from build123d import *

# Parameters (mm, degrees)
F1_DEPTH = 12.7
F3_DEPTH = 12.701


with BuildPart() as f1:
    # F0 (on Top) → F1 (new body)
    with BuildSketch(Plane.XY):
        with BuildLine():
            Line((-53.430256, 31.75), (-82.55, 31.75))
            ThreePointArc((-82.55, 31.75), (-87.040128, 29.890128), (-88.9, 25.4))
            Line((-88.9, 25.4), (-88.9, 15.330256))
            ThreePointArc((-88.9, 15.330256), (-88.416635, 12.900216), (-87.040128, 10.840128))
            Line((-87.040128, 10.840128), (-33.609872, -42.590128))
            ThreePointArc((-33.609872, -42.590128), (-31.549784, -43.966635), (-29.119744, -44.45))
            Line((-29.119744, -44.45), (41.819744, -44.45))
            ThreePointArc((41.819744, -44.45), (44.249784, -43.966635), (46.309872, -42.590128))
            Line((46.309872, -42.590128), (99.740128, 10.840128))
            ThreePointArc((99.740128, 10.840128), (101.116635, 12.900216), (101.6, 15.330256))
            Line((101.6, 15.330256), (101.6, 25.4))
            ThreePointArc((101.6, 25.4), (99.740128, 29.890128), (95.25, 31.75))
            Line((95.25, 31.75), (66.130256, 31.75))
            ThreePointArc((66.130256, 31.75), (63.700216, 31.266635), (61.640128, 29.890128))
            Line((61.640128, 29.890128), (59.009872, 27.259872))
            ThreePointArc((59.009872, 27.259872), (56.949784, 25.883365), (54.519744, 25.4))
            Line((54.519744, 25.4), (-41.819744, 25.4))
            ThreePointArc((-41.819744, 25.4), (-44.249784, 25.883365), (-46.309872, 27.259872))
            Line((-46.309872, 27.259872), (-48.940128, 29.890128))
            ThreePointArc((-48.940128, 29.890128), (-51.000216, 31.266635), (-53.430256, 31.75))
        make_face()
    extrude(amount=F1_DEPTH)

    # F2 (on face) → F3 (cut, through all)
    with BuildSketch(Plane.XY.offset(12.7)):
        with BuildLine():
            ThreePointArc((5.708911, 12.7), (4.121411, 12.274631), (2.95928, 11.1125))
            Line((2.95928, 11.1125), (-19.037765, -26.9875))
            ThreePointArc((-19.037765, -26.9875), (-19.037765, -30.1625), (-16.288134, -31.75))
            Line((-16.288134, -31.75), (28.988134, -31.75))
            ThreePointArc((28.988134, -31.75), (31.737765, -30.1625), (31.737765, -26.9875))
            Line((31.737765, -26.9875), (9.74072, 11.1125))
            ThreePointArc((9.74072, 11.1125), (8.578589, 12.274631), (6.991089, 12.7))
            Line((6.991089, 12.7), (5.708911, 12.7))
        make_face()
        with BuildLine():
            ThreePointArc((34.487395, 12.7), (31.737765, 11.1125), (31.737765, 7.9375))
            Line((31.737765, 7.9375), (46.923048, -18.364181))
            ThreePointArc((46.923048, -18.364181), (49.258258, -19.924519), (51.917742, -19.021745))
            Line((51.917742, -19.021745), (78.219424, 7.279936))
            ThreePointArc((78.219424, 7.279936), (78.907677, 10.74002), (75.97436, 12.7))
            Line((75.97436, 12.7), (34.487395, 12.7))
        make_face()
        with BuildLine():
            ThreePointArc((-63.27436, 12.7), (-66.207677, 10.74002), (-65.519424, 7.279936))
            Line((-65.519424, 7.279936), (-35.73135, -22.508137))
            ThreePointArc((-35.73135, -22.508137), (-33.071866, -23.410911), (-30.736656, -21.850573))
            Line((-30.736656, -21.850573), (-13.538503, 7.9375))
            ThreePointArc((-13.538503, 7.9375), (-13.538503, 11.1125), (-16.288134, 12.7))
            Line((-16.288134, 12.7), (-63.27436, 12.7))
        make_face()
    extrude(amount=-F3_DEPTH, mode=Mode.SUBTRACT)


solid = f1.part
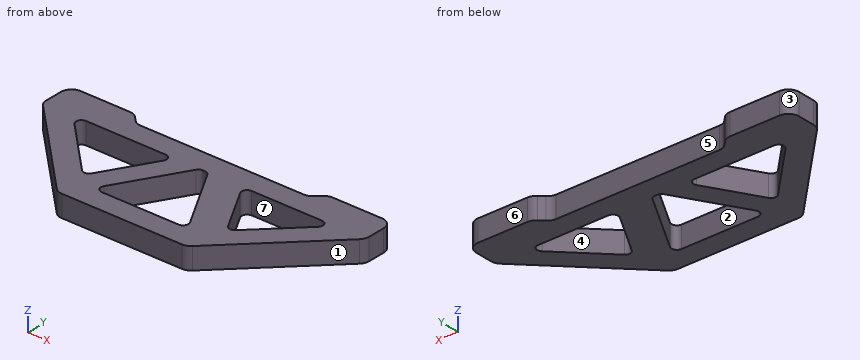
Geometry check sheet. Reference: the model listing, model coordinates, mm. Face numbers are marked on the shaded views. A direction names the side the tool comes from. Round coordinates to 2 decimals unless told otherwise and drop trailing zeros. Order: outer loops, then holes, each group sorted by start corner. A loop starts at its lowest first (then second) coordinate and runs counter-clockwise, first axis right, second up. Notation, with made-up numbers: M -10.75,8.25 L 16.25,8.25 A36 cw 16.25,43.25 Z; hole C 80,51 d10. An arc over 180 degrees is marked long. Answer in a Markdown table with one row per item. Add a question column.
Item 1: Sectioned sample at C-C, the plane z = 5. State how many separate pieces and enclosed holes the cut face has, plus the area to 3 significant figures.
Item 2: Set-up check for the marked faces 5, 6 and 7: record each of +Z, -Z, +X, -X, +Y, -Y from which the full face is reachable in a straight line by a thin tool's end or side.
Item 3: Draft check along Y on the marked faces 1, 2, 3 and 4. Enter one of: released by +Y, released by -Y, zero draft, split by the parting line, or undercut.
Item 4: Sectioned sample at A-A, the plane x = -58.5. Enter the section's corners in (y, z), plus the area to 3 significant figures.
Item 5: Sectioned sample at D-D, the plane x = -6. Enter the section's corners in (y, z), plus the area to 3 significant figures.
Item 6: Material ranges on L1, parallel to X at y = 5, z = 9; L2, parallel to X at y = -7, z = 7; L3, parallel to Y at x = -17, z = 10.75, recorded low to high. Write a range as [from, to].
Item 7: Sectioned sample at B-B, the plane y = -10.5. Enter the section's corners in (x, z), plus the area to 3 significant figures.
Item 8: Depth check by flat-ended pin: pin 1 Ø3 at (x, z) = (-16.5, 9) entering from +Y; pin 2 Ø6 at (y, z) = (-31, 5.5) entering from +X; pin 3 Ø4 at (x, z) = (-59, 3) entering from -Y; pin 4 Ø5 at (x, y) = (-13.5, 10.5) entering from +Z. Enter the tip coordinate at first touch or a pass-through.
Filled in:
| question | item | result |
|---|---|---|
| 1 | separate pieces | 1 |
| 1 | enclosed holes | 3 |
| 1 | area | 7,150 mm² |
| 2 | face 5 | +Z, -Z, +Y |
| 2 | face 6 | +Z, -Z, +X, -X, +Y |
| 2 | face 7 | +Z, -Z |
| 3 | face 1 | released by -Y |
| 3 | face 2 | undercut |
| 3 | face 3 | released by +Y |
| 3 | face 4 | undercut |
| 4 | outline | M -17.7,0 L 0.26,0 L 0.26,12.7 L -17.7,12.7 Z; M 12.7,0 L 31.75,0 L 31.75,12.7 L 12.7,12.7 Z |
| 4 | area | 470 mm² |
| 5 | outline | M -44.45,0 L -31.75,0 L -31.75,12.7 L -44.45,12.7 Z; M -4.41,0 L 25.4,0 L 25.4,12.7 L -4.41,12.7 Z |
| 5 | area | 540 mm² |
| 6 | L1 | x = [-81.2, -63.24], [-15.23, -0.57], [13.27, 33.43], [75.94, 93.9] |
| 6 | L2 | x = [-69.2, -51.24], [-22.16, -7.5], [20.2, 40.36], [63.94, 81.9] |
| 6 | L3 | y = [-44.45, -31.67], [-23.46, 1.94], [12.7, 25.4] |
| 7 | outline | M -65.7,0 L -47.74,0 L -47.74,12.7 L -65.7,12.7 Z; M -24.18,0 L -9.52,0 L -9.52,12.7 L -24.18,12.7 Z; M 22.22,0 L 42.38,0 L 42.38,12.7 L 22.22,12.7 Z; M 60.44,0 L 78.4,0 L 78.4,12.7 L 60.44,12.7 Z |
| 7 | area | 899 mm² |
| 8 | pin 1 | stops at y = 25.4 |
| 8 | pin 2 | stops at x = 60.9 |
| 8 | pin 3 | stops at y = -19.2 |
| 8 | pin 4 | stops at z = 12.7 |
